```python
from build123d import *

# Parameters (mm, degrees)
F2_DEPTH = 35.56
F0_R     = 10.16
F3_DEPTH = 76.2


# Not quite as in the source:
# - a feature names something its author has since deleted; it is built from what else it names


with BuildPart() as f2:
    # F1 (on Top) → F2 (new body)
    with BuildSketch(Plane.XY):
        with BuildLine():
            Line((0, 76.2), (-76.2, 76.2))
            Line((-76.2, 76.2), (-76.2, 10.16))
            ThreePointArc((-76.2, 10.16), (-73.2242048969, 2.9757951031), (-66.04, 0))
            Line((-66.04, 0), (-10.16, 0))
            ThreePointArc((-10.16, 0), (-2.9757951031, 2.9757951031), (0, 10.16))
            Line((0, 10.16), (0, 76.2))
        make_face()
    extrude(amount=F2_DEPTH)

    # F0 (on Right) → F3 (join)
    with BuildSketch(Plane.YZ):
        Polygon((76.2, 0), (111.76, 0), (147.32, 35.56), (147.32, 71.12), (111.76, 71.12), (76.2, 35.56), align=None)
        with Locations((93.98, 20.32)):
            Circle(F0_R, mode=Mode.SUBTRACT)
    extrude(amount=-F3_DEPTH)


solid = f2.part
```
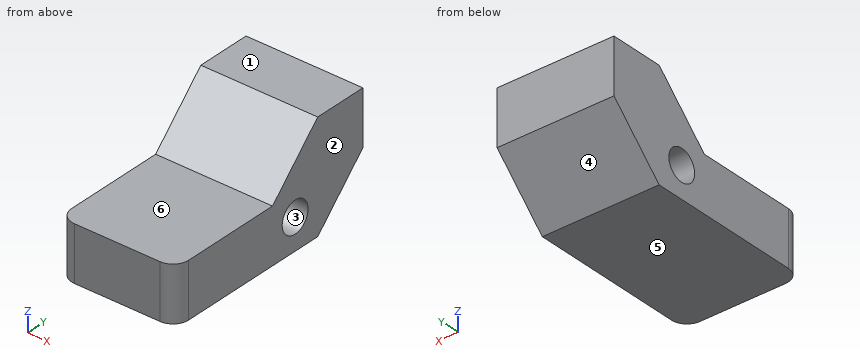
Here's how the part is built. I have some questions about the finished solid (model axes, mm). Face numbers are marked on the shaded views. A direction names the side the tool comes from. Give positions to 0.01 mm unless a question says otherwise; leave off trailing zeros. Order: outer loops, then holes, each group sorted by start corner. A loop starts at its lowest first (then second) coordinate and runs counter-clockwise, first axis right, second up. Notation, with made-up numbers: (55.25, 21) - (60.25, 21) arc R21 cw to (60.25, 43) - close; hole circle Ø2 at (21, -29). An arc over 180 degrees is marked (long way). Answer as a JSON object with one key per item and string values. Group by question number.
Item 1: Which directions (+Z, -Z, +X, -X, +Y, -Y) give clear straight access to the entire face, cutting with the end or side of a thin tool? Please do the marked faces 5 and 6.
Item 2: If we section it at C-C on x = -18.5: Please give me the cut outline in (y, z), and give its area (3 significant figures).
Item 3: If we section it at D-D on y = 115: Please give me the cut outline in (x, z), and give its area (3 significant figures).
Item 4: Please list where these lines run through material, in increasing order: probe 1 along Y at (x, z) = (-49, 20); probe 2 along Z at (x, y) = (-55.5, 93.98); probe 3 along Z at (x, y) = (-7, 49.5).
Item 5: For P1, Ø16.5, axis at y = 93.98, z = 20.32, coming from the -X side; P2, Ø4, axis at x = -59.5, z = 12.5, coming from the +Y side; P3, Ø10, axis at x = -42.5, z = 49, coming from the -Y side; P4, Ø23, axis at x = -51.5, y = 44, coming from the +Z side, each with a flat end and sliding along its axis, tell me the tip position at first contact or that it passes through.
Item 6: If we mould it in two halves opening along Z, with no side actions, what happens to the marked faces 1, 2, 3 and 4? For each: pulls with the +Z half, pulls with the -Z half, needs draft (parallel to the pull), parting line crosses it, or undercut.
Item 7: If we section it at B-B on y = 93.98: Please give me the cut outline in (x, z).
Item 8: If we section it at A-A on z = 20.32: Please give me the cut outline in (x, y).
Result set:
{
 "1": {"face 5": "-Z, +X, -X, +Y, -Y", "face 6": "+Z, +X, -X, -Y"},
 "2": {"outline": "(0, 0) - (111.76, 0) - (147.32, 35.56) - (147.32, 71.12) - (111.76, 71.12) - (76.2, 35.56) - (0, 35.56) - close; hole circle Ø20.32 at (93.98, 20.32)", "area": "6,180 mm²"},
 "3": {"outline": "(-76.2, 3.24) - (0, 3.24) - (0, 71.12) - (-76.2, 71.12) - close", "area": "5,170 mm²"},
 "4": {"probe 1": "0 to 83.83, 104.13 to 131.76", "probe 2": "0 to 10.16, 30.48 to 53.34", "probe 3": "0 to 35.56"},
 "5": {"P1": "through", "P2": "y = 126.26", "P3": "y = 84.64", "P4": "z = 35.56"},
 "6": {"face 1": "pulls with the +Z half", "face 2": "needs draft", "face 3": "undercut", "face 4": "pulls with the -Z half"},
 "7": {"outline": "(-76.2, 0) - (0, 0) - (0, 10.16) - (-76.2, 10.16) - close; (-76.2, 30.48) - (0, 30.48) - (0, 53.34) - (-76.2, 53.34) - close"},
 "8": {"outline": "(-76.2, 10.16) arc R10.16 ccw to (-66.04, 0) - (-10.16, 0) arc R10.16 ccw to (0, 10.16) - (0, 83.82) - (-76.2, 83.82) - close; (-76.2, 104.14) - (0, 104.14) - (0, 132.08) - (-76.2, 132.08) - close"}
}
